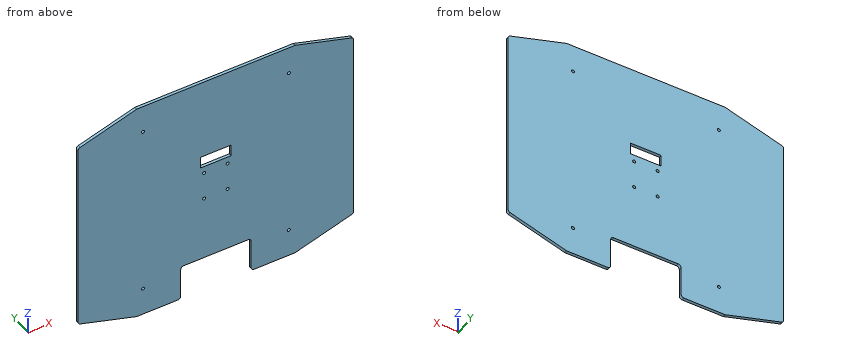
Autodesk Inventor part; units mm, degrees
ref_plane "YZ Plane" through (0, 0, 0) normal (1, 0, 0) x (0, 1, 0)
ref_plane "XZ Plane" through (0, 0, 0) normal (0, 1, 0) x (-1, 0, 0)
ref_plane "XY Plane" through (0, 0, 0) normal (0, 0, 1) x (1, 0, 0)
sketch "Sketch1" plane through (0, 0, 0) normal (0, 1, 0) x (-1, 0, 0)
  line L0 (149.225, -123.825) -> (-149.225, -123.825)
  line L1 (-149.225, -123.825) -> (-149.225, 123.825)
  line L2 (-149.225, 123.825) -> (149.225, 123.825)
  line L3 (149.225, 123.825) -> (149.225, -123.825)
  line L4 (149.225, -123.825) -> (-149.225, 123.825) construction
  line L5 (-149.225, -123.825) -> (149.225, 123.825) construction
  point P0 (0, 0)
  dimension "d0" = 298.45
  dimension "d1" = 247.65
extrude "Extrusion1" add sketch "Sketch1" along normal blind 3.175
sketch "Sketch2" plane through (0, 3.175, 0) normal (0, 1, 0) x (1, 0, 0)
  line L0 (149.225, 123.825) -> (-149.225, 123.825)
  line L1 (-149.225, 123.825) -> (-149.225, -123.825)
  line L2 (-149.225, -123.825) -> (149.225, -123.825)
  line L3 (149.225, -123.825) -> (149.225, 123.825)
  line L4 (-149.225, 104.775) -> (-85.725, 123.825)
  line L5 (85.725, 123.825) -> (149.225, 104.775)
  line L6 (149.225, -104.775) -> (85.725, -123.825)
  line L7 (-85.725, -123.825) -> (-149.225, -104.775)
  point P0 (0, 0)
  dimension "d4" = 19.05
  dimension "d5" = 19.05
  dimension "d6" = 19.05
  dimension "d7" = 19.05
  dimension "d8" = 63.5
  dimension "d9" = 63.5
  dimension "d10" = 63.5
extrude "Extrusion2" cut sketch "Sketch2" against normal blind 3.175 contours L3 L5 L0 | L4 L1 L0 | L3 L2 L6 | L7 L2 L1
sketch "Sketch3" plane through (0, 3.175, 0) normal (0, 1, 0) x (1, 0, 0)
  line L0 (85.725, 123.825) -> (-85.725, 123.825)
  line L1 (-38.1, 123.825) -> (38.1, 123.825)
  line L2 (38.1, 123.825) -> (38.1, 85.725)
  line L3 (38.1, 85.725) -> (-38.1, 85.725)
  line L4 (-38.1, 85.725) -> (-38.1, 123.825)
  point P0 (0, 0)
  point P1 (0, 85.725)
  dimension "d13" = 38.1
  dimension "d14" = 76.2
extrude "Extrusion3" cut sketch "Sketch3" against normal blind 3.175
fillet "Fillet1" radius 3.175 12 edges at (38.1, 1.5875, -85.725) (-38.1, 1.5875, -85.725) (38.1, 1.5875, -123.825) (-38.1, 1.5875, -123.825) (85.725, 1.5875, -123.825) (-85.725, 1.5875, -123.825) (-149.225, 1.5875, -104.775) (149.225, 1.5875, -104.775) (-149.225, 1.5875, 104.775) (-85.725, 1.5875, 123.825) (85.725, 1.5875, 123.825) (149.225, 1.5875, 104.775)
sketch "Sketch4" plane through (0, 3.175, 0) normal (0, 1, 0) x (1, 0, 0)
  point P0 (0, 0)
  point P1 (-78.9686, 93.5863)
  point P2 (-78.9686, -93.5863)
  point P3 (78.9686, -93.5863)
  point P4 (78.9686, 93.5863)
  dimension "d18" = 93.5863
  dimension "d19" = 93.5863
  dimension "d20" = 78.9686
  dimension "d21" = 78.9686
hole "Hole1" at (-78.9686, 3.175, -93.5863) at (-78.9686, 3.175, 93.5863) at (78.9686, 3.175, 93.5863) at (78.9686, 3.175, -93.5863) direction (0, -1, 0) diameter 3.302 end through all
sketch "Sketch5" plane through (0, 3.175, 0) normal (0, 1, 0) x (1, 0, 0)
  line L0 (-149.225, 102.4127) -> (-149.225, -102.4127)
  line L1 (149.225, -102.4127) -> (149.225, 102.4127)
  point P0 (0, 0)
  point P1 (-12.7, 15.24)
  point P2 (12.7, 15.24)
  point P3 (-12.7, -15.24)
  point P4 (12.7, -15.24)
  dimension "d38" = 25.4
  dimension "d39" = 25.4
  dimension "d40" = 30.48
  dimension "d44" = 15.24
  dimension "d45" = 15.24
  dimension "d46" = 12.7
  dimension "d47" = 12.7
  dimension "d48" = 12.7
hole "Hole3" at (-12.7, 3.175, -15.24) at (12.7, 3.175, -15.24) at (-12.7, 3.175, 15.24) at (12.7, 3.175, 15.24) direction (0, -1, 0) diameter 3.302 end through all
sketch "Sketch6" plane through (0, 3.175, 0) normal (0, 1, 0) x (1, 0, 0)
  line L0 (-16.51, -22.86) -> (16.51, -22.86)
  line L1 (16.51, -22.86) -> (16.51, -35.56)
  line L2 (16.51, -35.56) -> (-16.51, -35.56)
  line L3 (-16.51, -35.56) -> (-16.51, -22.86)
  point P0 (0, 0)
  dimension "d56" = 33.02
  dimension "d57" = 22.86
  dimension "d58" = 16.51
  dimension "d61" = 12.7
extrude "Extrusion4" cut sketch "Sketch6" against normal blind 25.4
properties part number "CoverPlate_CamMount"
Geometry: final body of the model. Coordinates: model frame, mm. Give positions to 0.01 mm unless a question says otherwise; leave off trailing zeros. Write each loop counter-clockwise with the first axis right and the second up, starting at its lowest first coordinate (ties: lowest second). Pieces come first, ordered by that corner, then holes. Notation, with made-up numbers: M 75.25,-1.75 L 112.25,-1.75 A21 ccw 112.25,27.25 Z; hole C -10.75,26 d9. An arc over 180 degrees is marked long. Answer in a Markdown table with one row per item. Add a question column.
(1) Section B-B on y = 0.55. State how many separate pieces and enclosed holes the cut face has, and give its area (3 significant figures).
(2) Section C-C on z = 109.5. Return loops of the section in (x, y) (3 decimals), and give its area (3 significant figures).
(3) Ray query, line 1 (X direction, y = 2.35, z = -92.5) (3 decimals); line 2 (Z direction, x = 0, y = 0.4) (3 decimals); line 3 (X direction, y = 1.05, z = -91) (3 decimals). Return the intervals inside material, ascending.
(4) First-contact query: pin 1 (1.6 mm diameter, centred on x = 6, y = 1, fed in from -Z) (3 decimals); pin 2 (1.5 mm diameter, centred on x = 105, y = 2.5, fed in from -Z); pin 3 (4 mm diameter, centred on x = -78.97, z = -93.59, fed in from +Y) (3 decimals). Flat tips, straight axial feed; report the tip coordinate or a pass-through.
(5) Section A-A on x = 5. Return loops of the section in (y, z) (3 decimals).
Result set:
| question | item | result |
|---|---|---|
| 1 | separate pieces | 1 |
| 1 | enclosed holes | 9 |
| 1 | area | 68,100 mm^2 |
| 2 | outline | M -133.475,0 L 133.475,0 L 133.475,3.175 L -133.475,3.175 Z |
| 2 | area | 848 mm^2 |
| 3 | line 1 | x = -149.225 to -80.212, -77.725 to -38.1, 38.1 to 77.725, 80.212 to 149.225 |
| 3 | line 2 | z = -85.725 to 22.86, 35.56 to 123.825 |
| 3 | line 3 | x = -149.225 to -38.1, 38.1 to 149.225 |
| 4 | pin 1 | stops at z = -85.725 |
| 4 | pin 2 | stops at z = -118.27 |
| 4 | pin 3 | stops at y = 3.175 |
| 5 | outline | M 0,-85.725 L 3.175,-85.725 L 3.175,22.86 L 0,22.86 Z; M 0,35.56 L 3.175,35.56 L 3.175,123.825 L 0,123.825 Z |
